```python
from build123d import *

# Parameters (mm, degrees)
EXTRUDE_1_DEPTH    = 30
HOLE_WIZARD_M4_1_D = 3.3


with BuildPart() as part:
    # 草图1 → 凸台-拉伸1 (new body)
    with BuildSketch(Plane(origin=(0, 0, 0), x_dir=(0, 0, -1), z_dir=(1, 0, 0))):
        Polygon((3.464101615, 0), (1.732050808, 3), (-1.732050808, 3), (-3.464101615, 0), (-1.732050808, -3), (1.732050808, -3), align=None)
    extrude(amount=EXTRUDE_1_DEPTH)

    # M4 螺纹孔1 (through all)
    with Locations(Plane.ZY):
        with Locations((0, 0)):
            Hole(HOLE_WIZARD_M4_1_D / 2)


solid = part.part
```
Build history of the part. All positions in model axes, mm. Give positions to 0.01 mm unless a question says otherwise; leave off trailing zeros. Loops run counter-clockwise (first coordinate to the right, second up) from the corner with the lowest first, then second, coordinate; pieces in that order, holes last. Notation, with made-up numbers: (57.5, 1.5) -> (105.5, 1.5) arc R16 cw to (105.5, 19.5) -> close; hole circle Ø9 at (34, 2.25). An arc over 180 degrees is marked (long way). One line per question, with ' | ' between items.
Q1. Cut at C-C, the plane y = -1. Write the cut outline in (x, z).
Filled sheet:
outline: (0, -2.89) -> (30, -2.89) -> (30, -1.31) -> (0, -1.31) -> close; (0, 1.31) -> (30, 1.31) -> (30, 2.89) -> (0, 2.89) -> close
Q2. Drop flat-ended pins along their axis: pin 1 (1.5 mm diameter, centred on x = 20, y = 1, fed in from -Z); pin 2 (2.5 mm diameter, centred on y = 0, z = 0, fed in from +X). Give the stop position or say it passes through.
Filled sheet:
pin 1: stops at z = -3.32 | pin 2: passes through
Q3. Cut at B-B, the plane z = 0. Write the cut outline in (x, y), plus the area to 3 significant figures.
Filled sheet:
outline: (0, -3) -> (30, -3) -> (30, -1.65) -> (0, -1.65) -> close; (0, 1.65) -> (30, 1.65) -> (30, 3) -> (0, 3) -> close | area: 81.0 mm²
Q4. Cut at D-D, the plane z = -2. Write the cut outline in (x, y), plus the area to 3 significant figures.
Filled sheet:
outline: (0, -2.54) -> (30, -2.54) -> (30, 2.54) -> (0, 2.54) -> close | area: 152 mm²
Q5. Cut at A-A, the plane x = 8.75. Write the cut outline in (y, z).
Filled sheet:
outline: (-3, -1.73) -> (0, -3.46) -> (3, -1.73) -> (3, 1.73) -> (0, 3.46) -> (-3, 1.73) -> close; hole circle Ø3.3 at (0, 0)
Q6. Drill centre lines: line 1 along Y through (x, z) = (23.25, 0); line 2 along Y through (x, z) = (10.5, -1.5); line 3 along Z through (x, y) = (7.5, -1.5). Where is each one in solid material? Low to high. Write a range as [from, to].
Filled sheet:
line 1: y = [-3, -1.65], [1.65, 3] | line 2: y = [-3, -0.69], [0.69, 3] | line 3: z = [-2.6, -0.69], [0.69, 2.6]
Q7. Pull direction Y, two halves, no side cores. Call faces 1 (the flat face through (30, 1.4, -1.5)), 2 (the cylindrical face through (15.21, 1.115, 1.216)), 3 (the flat face through (14.8, -1.5, 2.6)): pulls with the +Y half, pulls with the -Y half, needs draft (parallel to the pull), parting line crosses it, or undercut.
Filled sheet:
face 1: needs draft | face 2: undercut | face 3: pulls with the -Y half
